from build123d import *

# Parameters (mm, degrees)
SKETCH1_W               = 400
SKETCH1_H               = 200
BOSS_EXTRUDE1_DEPTH     = 300
CUT_EXTRUDE1_DEPTH      = 413.310562562
CUT_EXTRUDE1_DEPTH_BACK = 413.310562562
SHELL1_T                = -5
SKETCH3_W               = 430
SKETCH3_H               = 330
BOSS_EXTRUDE2_DEPTH     = 5
SHELL2_START            = 100
SHELL2_OUTLINE_W        = 390
SHELL2_OUTLINE_H        = 290
SHELL2_DEPTH            = 5
SKETCH5_W               = 130
SKETCH5_H               = 130
BOSS_EXTRUDE3_DEPTH     = 10


# Read off the part's stored shape, not the designer's step: Shell2
with BuildPart() as part:
    # Sketch1 → Boss-Extrude1 (new body)
    with BuildSketch(Plane.XY):
        Rectangle(SKETCH1_W, SKETCH1_H)
        Polygon((-50, -200), (50, -200), (200, -100), (-200, -100), align=None)
    extrude(amount=-BOSS_EXTRUDE1_DEPTH)

    # Sketch2 → Cut-Extrude1 (cut, two sides: drawn at the far end of the back side and taken through both)
    with BuildSketch(Plane(origin=(0, 0, 0), x_dir=(0, 0, -1), z_dir=(1, 0, 0)).offset(-CUT_EXTRUDE1_DEPTH_BACK)):
        Polygon((0, -100), (100, -200), (0, -200), align=None)
        Polygon((300, -100), (300, -200), (200, -200), align=None)
    extrude(amount=CUT_EXTRUDE1_DEPTH + CUT_EXTRUDE1_DEPTH_BACK, mode=Mode.SUBTRACT)

    # Shell1
    shell1_openings = [part.faces().sort_by_distance(p)[0] for p in [
        (0, -200, -150),
        (0, 100, -150),
    ]]
    offset(amount=SHELL1_T, openings=shell1_openings, kind=Kind.INTERSECTION)

    # Sketch3 → Boss-Extrude2 (add)
    with BuildSketch(Plane(origin=(0, 100, 0), x_dir=(1, 0, 0), z_dir=(0, 1, 0))):
        with Locations((0, 150)):
            Rectangle(SKETCH3_W, SKETCH3_H)
    extrude(amount=BOSS_EXTRUDE2_DEPTH)

    # Shell2 outline → Shell2 (cut)
    with BuildSketch(Plane(origin=(0, 0, 0), x_dir=(1, 0, 0), z_dir=(0, 1, 0)).offset(SHELL2_START)):
        with Locations((0, 150)):
            Rectangle(SHELL2_OUTLINE_W, SHELL2_OUTLINE_H)
    extrude(amount=SHELL2_DEPTH, mode=Mode.SUBTRACT)

    # Sketch5 → Boss-Extrude3 (add)
    with BuildSketch(Plane.XZ.offset(200)):
        with Locations((0, -150)):
            Rectangle(SKETCH5_W, SKETCH5_H)
    extrude(amount=BOSS_EXTRUDE3_DEPTH)


solid = part.part
Could you check a few things on this model? Use its own coordinates, in mm. A direction names the side the tool comes from. Coordinates: 2 decimals unless noted, no trailing zeros. Order: outer loops, then holes, each group sorted by start corner. A loop starts at its lowest first (then second) coordinate and runs counter-clockwise, first axis right, second up. Notation, with made-up numbers: (87.25, 33.25) -> (93.25, 33.25) arc R16 ccw to (93.25, 56.25) -> close; hole circle Ø11 at (39.5, -25.5). An arc over 180 degrees is marked (long way). One line per question, with ' | ' between items.
Q1. Imagine slicing it at A-A on y = 28. Please give me the cut outline in (x, z).
Return value:
outline: (-200, -300) -> (200, -300) -> (200, 0) -> (-200, 0) -> close; hole (-195, -295) -> (195, -295) -> (195, -5) -> (-195, -5) -> close
Q2. Thinking about a two-plate mould opening in X: for faces 4 (the face through (140.6, -139.6, -147.9)), 5 (the face through (-143, -138, -148)), 6 (the face through (-136.184, -136.535, -147.97)), 7 (the face through (-3, 1, 0)), which applies, pulls with the +X half, pulls with the -X half, needs draft (parallel to the pull), parting line crosses it, or undercut?
Return value:
face 4: pulls with the +X half | face 5: pulls with the -X half | face 6: undercut | face 7: needs draft
Q3. If I drill on L1, parallel to X at y = -76, z = -48; L2, parallel to Z at x = -64, y = -11.5; L3, parallel to X at y = -137, z = -224, over which ranges is the centre line in solid material (lowest first)?
Return value:
L1: -200 to -195, 195 to 200 | L2: -300 to -295, -5 to 0 | L3: -144.5 to -135.49, 135.49 to 144.5
Q4. Imagine slicing it at C-C on x = -23.5. Please give me the cut outline in (y, z), and give its area (3 significant figures).
Return value:
outline: (-210, -215) -> (-200, -215) -> (-200, -200) -> (-100, -300) -> (100, -300) -> (100, -315) -> (105, -315) -> (105, -295) -> (-97.93, -295) -> (-200, -192.93) -> (-200, -107.07) -> (-97.93, -5) -> (105, -5) -> (105, 15) -> (100, 15) -> (100, 0) -> (-100, 0) -> (-200, -100) -> (-200, -85) -> (-210, -85) -> close | area: 4,920 mm²
Q5. Imagine slicing it at B-B on z = -170.5. Please give me the cut outline in (x, y), and give its area (3 significant figures).
Return value:
outline: (-215, 100) -> (-200, 100) -> (-200, -100) -> (-50, -200) -> (-65, -200) -> (-65, -210) -> (65, -210) -> (65, -200) -> (50, -200) -> (200, -100) -> (200, 100) -> (215, 100) -> (215, 105) -> (195, 105) -> (195, -97.32) -> (40.99, -200) -> (-40.99, -200) -> (-195, -97.32) -> (-195, 105) -> (-215, 105) -> close | area: 5,310 mm²
Q6. On a 3-axis mill with a long thin cutter (end or side, diameter ignored), from which of +Z, -Z, +X, -X, +Y, -Y can I reach the whole of each face in a straight line? I mean faces 1 (the face through (-65, -205, -151)), 2 (the face through (-3, 2, -5)), 3 (the face through (-3, 1, -300)). Say none if no direction works.
Return value:
face 1: +Z, -Z, -X, -Y | face 2: +Y | face 3: -Z, +X, -X, -Y
Q7. Imagine slicing it at D-D on x = -94. Please give me the cut outline in (y, z), and give its area (3 significant figures).
Return value:
outline: (-170.67, -229.33) -> (-100, -300) -> (100, -300) -> (100, -315) -> (105, -315) -> (105, -295) -> (-97.93, -295) -> (-164.66, -228.27) -> (-164.66, -71.73) -> (-97.93, -5) -> (105, -5) -> (105, 15) -> (100, 15) -> (100, 0) -> (-100, 0) -> (-170.67, -70.67) -> close | area: 4,110 mm²
Q8. I'm going to push flat-ended pins straight in: P1, Ø2, axis at y = 7, z = -170.5, coming from the -X side; P2, Ø6, axis at x = 35.5, z = -133.5, coming from the +Y side; P3, Ø8, axis at x = -8.5, y = -204, coming from the +Z side. Where does each tip first touch, or does it pass through?
Return value:
P1: x = -200 | P2: y = -200 | P3: z = -85
